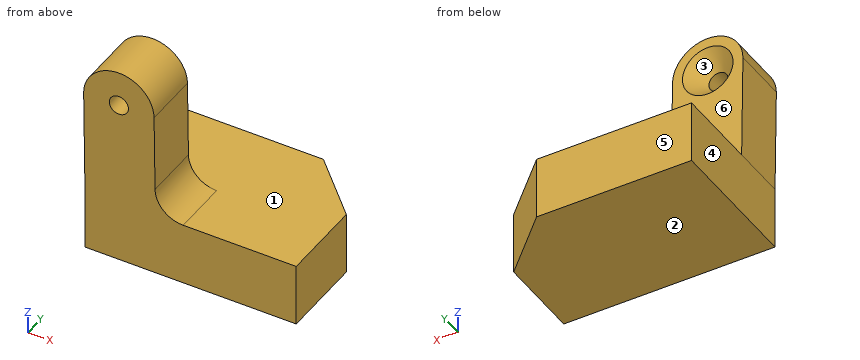
from build123d import *

# Parameters (mm, degrees)
F1_DEPTH       = 25.4
F2_DEPTH       = 15.24
F3_D           = 3.4544
F3_START       = 15.24
F3_CSINK_D     = 9.1186
F3_CSINK_ANGLE = 82
F4_R           = 5.08
F5_SIZE        = 10.16


with BuildPart() as f1:
    # F0 (on Front) → F1 (new body)
    with BuildSketch(Plane.XZ):
        Polygon((19.05, -5.6587588522), (19.05, 5.6587588522), (-6.35, 5.6587588522), (-19.05, 5.6587588522), (-19.05, -5.6587588522), align=None)
        with BuildLine():
            Line((-19.05, 5.6587588522), (-6.35, 5.6587588522))
            Line((-6.35, 5.6587588522), (-6.5872897774, 24.7072809356))
            ThreePointArc((-6.5872897774, 24.7072809356), (-12.9367971385, 30.9781843431), (-19.2863044996, 24.7072809356))
            Line((-19.2863044996, 24.7072809356), (-19.05, 5.6587588522))
        make_face()
    extrude(amount=F1_DEPTH)

    # F0 (on Front) → F2 (cut)
    with BuildSketch(Plane.XZ):
        with BuildLine():
            Line((-19.05, 5.6587588522), (-6.35, 5.6587588522))
            Line((-6.35, 5.6587588522), (-6.5872897774, 24.7072809356))
            ThreePointArc((-6.5872897774, 24.7072809356), (-12.9367971385, 30.9781843431), (-19.2863044996, 24.7072809356))
            Line((-19.2863044996, 24.7072809356), (-19.05, 5.6587588522))
        make_face()
    extrude(amount=F2_DEPTH, mode=Mode.SUBTRACT)

    # F3 (through all)
    # its depths count from where the whole tool has entered the part; down to there all is cleared
    with Locations(Plane(origin=(0, 0, 0), x_dir=(1, 0, 0), z_dir=(0, 1, 0)).offset(-F3_START)):
        with Locations((-12.9367971385, -24.6281843431)):
            CounterSinkHole(F3_D / 2, F3_CSINK_D / 2, counter_sink_angle=F3_CSINK_ANGLE)

    # F4
    f4_edges = [f1.edges().sort_by_distance(p)[0] for p in [
        (-6.35, -20.32, 5.658759),
    ]]
    fillet(f4_edges, radius=F4_R)

    # F5
    f5_edges = [f1.edges().sort_by_distance(p)[0] for p in [
        (19.05, 0, 0),
    ]]
    chamfer(f5_edges, length=F5_SIZE)


solid = f1.part
For this review, take the finished solid that the model builds, in its own axes (mm). Face numbers are marked on the shaded views. A direction names the side the tool comes from. Give positions to 0.01 mm unless a question says otherwise; leave off trailing zeros. Write each loop counter-clockwise with the first axis right and the second up, starting at its lowest first coordinate (ties: lowest second). Pieces come first, ordered by that corner, then holes. Notation, with made-up numbers: (83, -15) -> (105, -15) arc R16 ccw to (105, -4) -> close; hole circle Ø1 at (54, 52.5). An arc over 180 degrees is marked (long way). Use CSV: the item, a comma, the result in double quotes.
Q1. Take a section at D-D, the plane y = -3.25. Write out the cut boundary in (x, z), then the cut area to 3 significant figures.
Conclusion:
outline,"(-19.05, -5.66) -> (12.14, -5.66) -> (12.14, 5.66) -> (-19.05, 5.66) -> close"
area,"353 mm2"
Q2. Take a section at C-C, the plane x = 4. Write out the cut boundary in (y, z).
Conclusion:
outline,"(-25.4, -5.66) -> (0, -5.66) -> (0, 5.66) -> (-25.4, 5.66) -> close"
Q3. Take a section at B-B, the plane z = 3. Write out the cut boundary in (x, y), then the cut area to 3 significant figures.
Conclusion:
outline,"(-19.05, -25.4) -> (19.05, -25.4) -> (19.05, -10.16) -> (8.89, 0) -> (-19.05, 0) -> close"
area,"916 mm2"
Q4. For P1, Ø5, axis at y = -21.5, z = 21, coming from the +X side; P2, Ø6, axis at x = 15, y = -19, coming from the +Z side; P3, Ø3.5, axis at y = -13.5, z = -0.5, coming from the -X side, all flat-tipped, find the tip position at first contact; note any pin that passes through.
Conclusion:
P1,"x = -6.51"
P2,"z = 5.66"
P3,"x = -19.05"
Q5. Tool access review of the marked faces 4, 5 and 6: name each direction out of +Z, -Z, +X, -X, +Y, -Y from which nothing blocks a thin tool from reaching the whole face with its end or side.
Conclusion:
face 4,"-Z, -X, +Y, -Y"
face 5,"+Z, -Z, +X, -X, +Y"
face 6,"+Z, +X, -X, +Y"
Q6. To check wall thickness, follow probe 1 along Z at (x, y) = (-10.5, -6.5); probe 2 along X at (y, z) = (-19.25, 1.5); probe 3 along X at (y, z) = (-17.25, 26.5). State the ranges of each line that lie inside material, in increasing order. Write a range as [from, to].
Conclusion:
probe 1,"[-5.66, 5.66]"
probe 2,"[-19.05, 19.05]"
probe 3,"[-19, -15.04], [-10.84, -6.87]"
Q7. Take a section at A-A, the plane y = -24. Write out the cut boundary in (x, z), then the cut area to 3 significant figures.
Conclusion:
outline,"(-19.29, 24.71) -> (-19.05, 5.66) -> (-19.05, -5.66) -> (19.05, -5.66) -> (19.05, 5.66) -> (-1.33, 5.66) arc R5.08 cw to (-6.41, 10.68) -> (-6.59, 24.71) arc R6.35 ccw to start; hole circle Ø3.45 at (-12.94, 24.63)"
area,"731 mm2"
Q8. Mouldability with a two-part tool opening along Z and no side actions: class the marked faces 1, 2 and 3 as pulls with the +Z half, pulls with the -Z half, needs draft (parallel to the pull), parting line crosses it, or undercut.
Conclusion:
face 1,"pulls with the +Z half"
face 2,"pulls with the -Z half"
face 3,"undercut"
